Verification items for the finished model (mm, model axes). Coordinates: 2 decimals unless noted, no trailing zeros. Write each loop counter-clockwise with the first axis right and the second up, starting at its lowest first coordinate (ties: lowest second). Pieces come first, ordered by that corner, then holes. Notation, with made-up numbers: M 17,72.5 L 59,72.5 A19 ccw 59,90.5 Z; hole C 89.25,-20 d9. An arc over 180 degrees is marked long. One line per item, written item: value.
```python
from build123d import *

# Parameters (mm, degrees)
SKETCH_1_W      = 27
SKETCH_1_H      = 18.6
SKETCH_1_R      = 2.7
EXTRUDE_1_DEPTH = 5
FILLET_2_R      = 1
FILLET_3_R      = 1


with BuildPart() as part:
    # 草图1 → 凸台-拉伸1 (new body)
    with BuildSketch(Plane(origin=(0, 0, 0), x_dir=(1, 0, 0), z_dir=(0, 1, 0))):
        with Locations((13.5, -9.3)):
            Rectangle(SKETCH_1_W, SKETCH_1_H)
        with Locations(Location((5.75, -10, 0), (0, 0, 270))):
            Circle(SKETCH_1_R, mode=Mode.SUBTRACT)
        with Locations(Location((21.25, -10, 0), (0, 0, 270))):
            Circle(SKETCH_1_R, mode=Mode.SUBTRACT)
    extrude(amount=EXTRUDE_1_DEPTH)

    # 圆角2
    fillet_2_edges = [part.edges().sort_by_distance(p)[0] for p in [
        (0, 2.5, 0),
        (27, 2.5, 0),
        (27, 2.5, 18.6),
        (0, 2.5, 18.6),
    ]]
    fillet(fillet_2_edges, radius=FILLET_2_R)

    # 圆角3
    fillet_3_edges = [part.edges().sort_by_distance(p)[0] for p in [
        (5.75, 5, 7.3),
        (21.25, 5, 7.3),
        (0, 5, 9.3),
        (13.5, 5, 0),
        (13.5, 5, 18.6),
        (27, 5, 9.3),
        (26.707106781, 5, 18.307106781),
        (0.292893219, 5, 18.307106781),
        (26.707106781, 5, 0.292893219),
        (0.292893219, 5, 0.292893219),
    ]]
    fillet(fillet_3_edges, radius=FILLET_3_R)


solid = part.part
```
Item 1: Scan lines: line 1 (X direction, y = 2.6, z = 10); line 2 (X direction, y = 4.4, z = 10.5); line 3 (Z direction, x = 10, y = 4.5). Record each from-to range of solid material in increasing order.
The answers:
line 1: x = 0 to 3.05, 8.45 to 18.55, 23.95 to 27
line 2: x = 0.08 to 3.01, 8.49 to 18.51, 23.99 to 26.92
line 3: z = 0.13 to 18.47
Item 2: Draft check along X on faces 1 (the face through (26.715, 4.699, 9.416)), 2 (the face through (13, 2, 18.6)), 3 (the face through (23.927, 1.972, 9.649)), 4 (the face through (0, 2, 9)). Enter one of: released by +X, released by -X, zero draft, split by the parting line, or undercut.
The answers:
face 1: released by +X
face 2: zero draft
face 3: undercut
face 4: released by -X
Item 3: Cross-section at B-B, the plane y = 0.5. Enter the section's corners in (x, z), and give its area (3 significant figures).
The answers:
outline: M 0,1 A1 ccw 1,0 L 26,0 A1 ccw 27,1 L 27,17.6 A1 ccw 26,18.6 L 1,18.6 A1 ccw 0,17.6 Z; hole C 5.75,10 d5.4; hole C 21.25,10 d5.4
area: 456 mm²
Item 4: Cross-section at C-C, the plane z = 10. Enter the section's corners in (x, y).
The answers:
outline: M 0,0 L 3.05,0 L 3.05,4 A1 ccw 2.05,5 L 1,5 A1 ccw 0,4 Z; M 8.45,0 L 18.55,0 L 18.55,4 A1 ccw 17.55,5 L 9.45,5 A1 ccw 8.45,4 Z; M 23.95,0 L 27,0 L 27,4 A1 ccw 26,5 L 24.95,5 A1 ccw 23.95,4 Z
Item 5: Cross-section at A-A, the plane x = 21.25. Enter the section's corners in (y, z), and give its area (3 significant figures).
The answers:
outline: M 0,0 L 4,0 A1 ccw 5,1 L 5,6.3 A1 ccw 4,7.3 L 0,7.3 Z; M 0,12.7 L 4,12.7 A1 ccw 5,13.7 L 5,17.6 A1 ccw 4,18.6 L 0,18.6 Z
area: 65.1 mm²
Item 6: Go/stop test with a flat-tipped pin: P1, Ø4.5, axis at x = 21.25, z = 10, coming from the +Y side. Record where the tip stops, or that it passes through.
The answers:
P1: passes through
Item 7: Cross-section at D-D, the plane z = 12.25. Give the number of separate pieces and of enclosed holes in the cut face, and give its area (3 significant figures).
The answers:
separate pieces: 3
enclosed holes: 0
area: 103 mm²
